The listing builds one solid part. Answer for the finished solid, in the listing's coordinates (mm). Round coordinates to 2 decimals unless told otherwise and drop trailing zeros. Loops run counter-clockwise (first coordinate to the right, second up) from the corner with the lowest first, then second, coordinate; pieces in that order, holes last. Notation, with made-up numbers: M 58.25,22.25 L 106.25,22.25 A29 ccw 106.25,43.25 Z; hole C -35,-39 d1. An arc over 180 degrees is marked long. Put each result on its own line as item: value. Start each with the question number.
(1) Section C-C, the plane y = 11.5 is taken. Determine the outline of the cut face in (x, z), then the cut area to 3 significant figures.
(2) Section B-B, the plane x = 0 is taken. Determine the outline of the cut face in (y, z), then the cut area to 3 significant figures.
(3) Straight lines are drawn through the part: line 1 (X direction, y = -0.1, z = 0); line 2 (Y direction, x = -7, z = -24); line 3 (X direction, y = 1.5, z = 0). For each, find the intervals that lie inside material, in ascending order.
(4) Section A-A, the plane z = 0 is taken. Determine the outline of the cut face in (x, y).
(5) Flat-ended cylindrical pins translate along their axes: P1, Ø4, axis at y = 10.5, z = -9, coming from the -X side; P2, Ø2, axis at x = -15, z = -14.5, coming from the -Y side; P3, Ø2, axis at y = 6, z = -1.5, coming from the +X side. Find the tip coordinate at first contact, or state that the pin passes through.
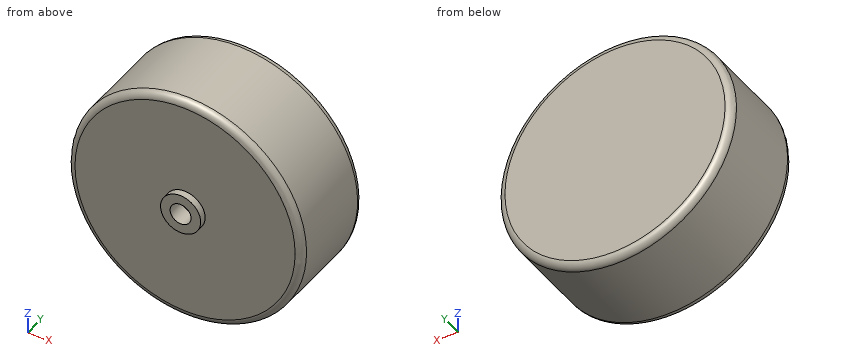
```python
from build123d import *

# Parameters (mm, degrees)
ESBO_O1_R                = 33.5
RESSALTO_EXTRUS_O1_DEPTH = 27
FILETE1_R                = 2
ESBO_O2_R                = 5.75
RESSALTO_EXTRUS_O2_DEPTH = 2
ESBO_O3_R                = 3
CORTE_EXTRUS_O1_DEPTH    = 5


with BuildPart() as part:
    # Esboço1 → Ressalto-extrusão1 (new body)
    with BuildSketch(Plane(origin=(0, 0, 0), x_dir=(1, 0, 0), z_dir=(0, 1, 0))):
        with Locations(Location((0, 0, 0), (0, 0, 270))):
            Circle(ESBO_O1_R)
    extrude(amount=RESSALTO_EXTRUS_O1_DEPTH)

    # Filete1
    filete1_edges = [part.edges().sort_by_distance(p)[0] for p in [
        (0, 0, -33.5),
        (0, 27, -33.5),
    ]]
    fillet(filete1_edges, radius=FILETE1_R)

    # Esboço2 → Ressalto-extrusão2 (add)
    with BuildSketch(Plane(origin=(0, 0, 0), x_dir=(-1, 0, 0), z_dir=(0, -1, 0))):
        with Locations(Location((0, 0, 0), (0, 0, 270))):
            Circle(ESBO_O2_R)
    extrude(amount=RESSALTO_EXTRUS_O2_DEPTH)

    # Esboço3 → Corte-extrusão1 (cut)
    with BuildSketch(Plane.XZ.offset(2)):
        with Locations(Location((0, 0, 0), (0, 0, 270))):
            Circle(ESBO_O3_R)
    extrude(amount=-CORTE_EXTRUS_O1_DEPTH, mode=Mode.SUBTRACT)


solid = part.part
```
Recorded:
1. outline: C 0,0 d67
1. area: 3,530 mm²
2. outline: M -2,-5.75 L 0,-5.75 L 0,-31.5 A2 ccw 2,-33.5 L 25,-33.5 A2 ccw 27,-31.5 L 27,31.5 A2 ccw 25,33.5 L 2,33.5 A2 ccw 0,31.5 L 0,5.75 L -2,5.75 L -2,3 L 3,3 L 3,-3 L -2,-3 Z
2. area: 1,800 mm²
3. line 1: x = -5.75 to -3, 3 to 5.75
3. line 2: y = 0 to 27
3. line 3: x = -33.44 to -3, 3 to 33.44
4. outline: M -33.5,2 A2 ccw -31.5,0 L -5.75,0 L -5.75,-2 L -3,-2 L -3,3 L 3,3 L 3,-2 L 5.75,-2 L 5.75,0 L 31.5,0 A2 ccw 33.5,2 L 33.5,25 A2 ccw 31.5,27 L -31.5,27 A2 ccw -33.5,25 Z
5. P1: stops at x = -32.76
5. P2: stops at y = 0
5. P3: stops at x = 33.5
